For this review, use the dimensioned drawing (mm, ordinates from the lowest corner) and the shaded views. Give positions to 0.01 mm unless a question says otherwise; leave off trailing zeros. Write each loop counter-clockwise with the first axis right and the second up, starting at its lowest first coordinate (ties: lowest second). Pieces come first, ordered by that corner, then holes. Notation, with made-up numbers: (74, 45.25) -> (79, 45.25) arc R32 cw to (79, 80.25) -> close; hole circle Ø6 at (46, -0.75). An arc over 180 degrees is marked (long way). Write each question's results on one line, items separated by ' | '. Start each with the question number.
(1) Clearance check with flat-ended pins moving along their axes: pin 1 (3 mm diameter, centred on x = 72.5, y = 4, fed in from +Z); pin 2 (1 mm diameter, centred on y = 2.5, z = 56.5, fed in from +X); pin 3 (3 mm diameter, centred on y = 3, z = 107, fed in from -X). State where each tip first meets the part, or that it passes through.
(2) Take a section at A-A (x = 71.5). State the section outline as (y, z) points, plus the area to 3 significant figures.
(3) To check wall thickness, follow probe 1 along Z at (x, y) = (71.5, 4); probe 2 along X at (y, z) = (3, 105). State the ranges of each line that lie inside material, in increasing order.
(4) Take a section at B-B (y = 3.5). State the section outline as (x, z) points.
(5) Take a section at C-C (z = 48). State the section outline as (x, y) points, plus the area to 3 significant figures.
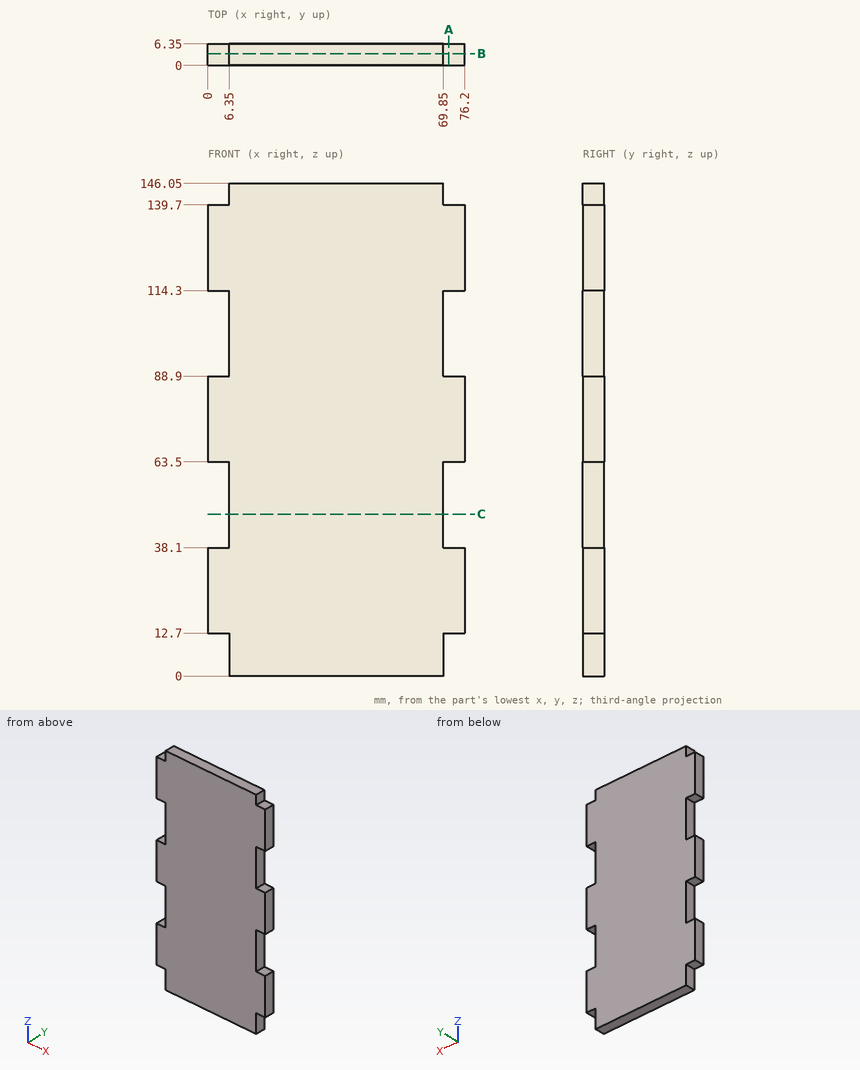
Report:
1) pin 1: z = 139.7 | pin 2: x = 69.85 | pin 3: x = 6.35
2) outline: (0, 12.7) -> (6.35, 12.7) -> (6.35, 38.1) -> (0, 38.1) -> close; (0, 63.5) -> (6.35, 63.5) -> (6.35, 88.9) -> (0, 88.9) -> close; (0, 114.3) -> (6.35, 114.3) -> (6.35, 139.7) -> (0, 139.7) -> close | area: 484 mm2
3) probe 1: 12.7 to 38.1, 63.5 to 88.9, 114.3 to 139.7 | probe 2: 6.35 to 69.85
4) outline: (0, 12.7) -> (6.35, 12.7) -> (6.35, 0) -> (69.85, 0) -> (69.85, 12.7) -> (76.2, 12.7) -> (76.2, 38.1) -> (69.85, 38.1) -> (69.85, 63.5) -> (76.2, 63.5) -> (76.2, 88.9) -> (69.85, 88.9) -> (69.85, 114.3) -> (76.2, 114.3) -> (76.2, 139.7) -> (69.85, 139.7) -> (69.85, 146.05) -> (6.35, 146.05) -> (6.35, 139.7) -> (0, 139.7) -> (0, 114.3) -> (6.35, 114.3) -> (6.35, 88.9) -> (0, 88.9) -> (0, 63.5) -> (6.35, 63.5) -> (6.35, 38.1) -> (0, 38.1) -> close
5) outline: (6.35, 0) -> (69.85, 0) -> (69.85, 6.35) -> (6.35, 6.35) -> close | area: 403 mm2
